Model file for the job. Use its own axes, mm. Give positions to 0.01 mm unless a question says otherwise; leave off trailing zeros. Order: outer loops, then holes, each group sorted by start corner. A loop starts at its lowest first (then second) coordinate and runs counter-clockwise, first axis right, second up. Notation, with made-up numbers: (16, 27) - (36, 27) arc R25 cw to (36, 53) - close; hole circle Ø8 at (25.25, 76). An arc over 180 degrees is marked (long way). Use CSV: the item, a comma, the result in double quotes. Start each with the question number.
(1) Band-saw the part on D-D, the plane x = 60.5. Give the cut face in (y, z).
(2) Band-saw the part on B-B, the plane x = -1.5. Give the cut face in (y, z).
(3) Probe L1, parallel to X at y = 4.6, z = 61; L2, parallel to X at y = 4.9, z = 44.5; L3, parallel to Z at x = -8, y = 5.15. List the from-to ranges inside material, lowest first.
(4) Band-saw the part on C-C, the plane y = 3.45. Count the separate pieces of the cut face and the enclosed holes in it, then the cut area to 3 significant figures.
(5) Band-saw the part on A-A, the plane z = 66.5. Give the cut face in (x, y).
(6) Drop flat-ended pins along their axis: pin 1 Ø3 at (y, z) = (3, -82.5) entering from -X; pin 2 Ø1.8 at (x, y) = (-22, 4) entering from +Z. Give the stop position or say it passes through.
from build123d import *

# Parameters (mm, degrees)
BOSS_EXTRUDE1_DEPTH = 6
SKETCH2_W           = 10
SKETCH2_H           = 10
CUT_EXTRUDE1_DEPTH  = 6
SKETCH4_W           = 40
SKETCH4_H           = 6
SKETCH4_W_2         = 6
SKETCH4_H_2         = 40
SKETCH4_H_3         = 15
CUT_EXTRUDE2_DEPTH  = 6


with BuildPart() as part:
    # Sketch1 → Boss-Extrude1 (new body)
    with BuildSketch(Plane(origin=(0, 0, 0), x_dir=(1, 0, 0), z_dir=(0, 1, 0))):
        Polygon((-94, 86), (-74, 86), (-74, 80), (-54, 80), (-54, 86), (-34, 86), (-34, 80), (-14, 80), (-14, 86), (6, 86), (6, 80), (26, 80), (26, 86), (46, 86), (46, 80), (66, 80), (66, 86), (86, 86), (86, 80), (114, 80), (114, -80), (86, -80), (86, -86), (66, -86), (66, -80), (46, -80), (46, -86), (26, -86), (26, -80), (6, -80), (6, -86), (-14, -86), (-14, -80), (-34, -80), (-34, -86), (-54, -86), (-54, -80), (-74, -80), (-74, -86), (-94, -86), (-94, -80), (-114, -80), (-114, 80), (-94, 80), align=None)
    extrude(amount=BOSS_EXTRUDE1_DEPTH)

    # Sketch2 → Cut-Extrude1 (cut)
    with BuildSketch(Plane(origin=(0, 0, 0), x_dir=(1, 0, 0), z_dir=(0, 1, 0))):
        with Locations((-99, 59)):
            Rectangle(SKETCH2_W, SKETCH2_H)
        with Locations((99, 59)):
            Rectangle(SKETCH2_W, SKETCH2_H)
        with Locations((99, -59)):
            Rectangle(SKETCH2_W, SKETCH2_H)
        with Locations((-99, -59)):
            Rectangle(SKETCH2_W, SKETCH2_H)
    extrude(amount=CUT_EXTRUDE1_DEPTH, mode=Mode.SUBTRACT)

    # Sketch4 → Cut-Extrude2 (cut)
    with BuildSketch(Plane(origin=(0, 6, 0), x_dir=(1, 0, 0), z_dir=(0, 1, 0))):
        with Locations((0, -13)):
            Rectangle(SKETCH4_W, SKETCH4_H)
        with Locations((0, -87)):
            Rectangle(SKETCH4_W, SKETCH4_H)
        with Locations((-37, -50)):
            Rectangle(SKETCH4_W_2, SKETCH4_H_2)
        with Locations((37, -50)):
            Rectangle(SKETCH4_W_2, SKETCH4_H_2)
        with Locations((-27, 62.5)):
            Rectangle(SKETCH4_W_2, SKETCH4_H_3)
        with Locations((27, 62.5)):
            Rectangle(SKETCH4_W_2, SKETCH4_H_3)
    extrude(amount=-CUT_EXTRUDE2_DEPTH, mode=Mode.SUBTRACT)


solid = part.part
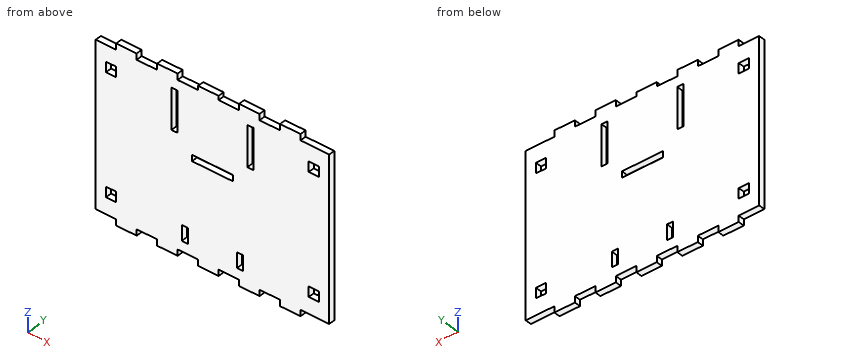
Answer block:
1,outline,"(0, -80) - (6, -80) - (6, 80) - (0, 80) - close"
2,outline,"(0, -86) - (6, -86) - (6, 10) - (0, 10) - close; (0, 16) - (6, 16) - (6, 84) - (0, 84) - close"
3,L1,"x = -114 to -104, -94 to -40, -34 to 34, 40 to 94, 104 to 114"
3,L2,"x = -114 to -40, -34 to 34, 40 to 114"
3,L3,"z = -86 to 10, 16 to 84"
4,separate pieces,"1"
4,enclosed holes,"9"
4,area,"36,300 mm2"
5,outline,"(-114, 0) - (-40, 0) - (-40, 6) - (-114, 6) - close; (-34, 0) - (34, 0) - (34, 6) - (-34, 6) - close; (40, 0) - (114, 0) - (114, 6) - (40, 6) - close"
6,pin 1,"stops at x = -94"
6,pin 2,"stops at z = 80"
